from build123d import *

# Parameters (mm, degrees)
BOSS_EXTRUDE1_DEPTH      = 96
SKETCH3_W                = 68
SKETCH3_H                = 10
CUT_EXTRUDE1_DEPTH       = 96
SKETCH6_W                = 5.25
SKETCH6_H                = 36
BOSS_EXTRUDE3_DEPTH      = 7
BOSS_EXTRUDE3_DEPTH_BACK = 103
SKETCH8_W                = 5.25
SKETCH8_H                = 7
BOSS_EXTRUDE4_DEPTH      = 4
SKETCH10_W               = 5.25
SKETCH10_H               = 7
BOSS_EXTRUDE5_DEPTH      = 4
SKETCH11_W               = 96
SKETCH11_H               = 36
CUT_EXTRUDE2_DEPTH       = 101
SKETCH12_R               = 1.85
CUT_EXTRUDE3_DEPTH       = 111
SKETCH13_W               = 96
SKETCH13_H               = 3.5
CUT_EXTRUDE4_DEPTH       = 10
SKETCH14_W               = 1
SKETCH14_H               = 13.753189639
CUT_EXTRUDE5_DEPTH       = 10
SKETCH15_W               = 25
SKETCH15_H               = 24
BOSS_EXTRUDE6_DEPTH      = 5
SKETCH16_W               = 22
SKETCH16_H               = 24
CUT_EXTRUDE6_DEPTH       = 3


with BuildPart() as part:
    # Sketch1 → Boss-Extrude1 (new body)
    with BuildSketch(Plane.XY):
        Polygon((2.5, 3), (5, 3), (5, -3), (-5, -3), (-5, 3), (-2.5, 3), (-2.5, 7), (-33, 7), (-33, 15.720359308), (-29, 15.720359308), (-29, 11), (29, 11), (29, 17.148290328), (33, 17.148290328), (33, 7), (2.5, 7), align=None)
    extrude(amount=-BOSS_EXTRUDE1_DEPTH)

    # Sketch3 → Cut-Extrude1 (cut)
    with BuildSketch(Plane.ZY.offset(5)):
        with Locations((-48, 2)):
            Rectangle(SKETCH3_W, SKETCH3_H)
    extrude(amount=-CUT_EXTRUDE1_DEPTH, mode=Mode.SUBTRACT)

    # Sketch6 → Boss-Extrude3 (add, two sides)
    with BuildSketch(Plane.XY) as boss_extrude3_sk:
        with Locations((14.625, -11)):
            Rectangle(SKETCH6_W, SKETCH6_H)
    extrude(amount=BOSS_EXTRUDE3_DEPTH)
    extrude(boss_extrude3_sk.sketch, amount=-BOSS_EXTRUDE3_DEPTH_BACK)

    # Sketch8 → Boss-Extrude4 (add)
    with BuildSketch(Plane(origin=(0, 7, 0), x_dir=(1, 0, 0), z_dir=(0, 1, 0))):
        with Locations((14.625, 99.5)):
            Rectangle(SKETCH8_W, SKETCH8_H)
    extrude(amount=BOSS_EXTRUDE4_DEPTH)

    # Sketch10 → Boss-Extrude5 (add)
    with BuildSketch(Plane(origin=(0, 7, 0), x_dir=(1, 0, 0), z_dir=(0, 1, 0))):
        with Locations((14.625, -3.5)):
            Rectangle(SKETCH10_W, SKETCH10_H)
    extrude(amount=BOSS_EXTRUDE5_DEPTH)

    # Sketch11 → Cut-Extrude2 (cut)
    with BuildSketch(Plane.ZY.offset(-12)):
        with Locations((-48, -11)):
            Rectangle(SKETCH11_W, SKETCH11_H)
    extrude(amount=-CUT_EXTRUDE2_DEPTH, mode=Mode.SUBTRACT)

    # Sketch12 → Cut-Extrude3 (cut, through all)
    with BuildSketch(Plane.XY.offset(7)):
        with Locations((14.5, -25.3)):
            Circle(SKETCH12_R)
        with Locations((14.5, -9.6)):
            Circle(SKETCH12_R)
    extrude(amount=-CUT_EXTRUDE3_DEPTH, mode=Mode.SUBTRACT)

    # Sketch13 → Cut-Extrude4 (cut)
    with BuildSketch(Plane.ZY.offset(33)):
        with Locations((-48, 13.970359308)):
            Rectangle(SKETCH13_W, SKETCH13_H)
    extrude(amount=-CUT_EXTRUDE4_DEPTH, mode=Mode.SUBTRACT)

    # Sketch14 → Cut-Extrude5 (cut)
    with BuildSketch(Plane.ZY.offset(-12)):
        with Locations((0.5, 0.12340518)):
            Rectangle(SKETCH14_W, SKETCH14_H)
        with Locations((-96.5, 0.12340518)):
            Rectangle(SKETCH14_W, SKETCH14_H)
    extrude(amount=-CUT_EXTRUDE5_DEPTH, mode=Mode.SUBTRACT)

    # Sketch15 → Boss-Extrude6 (add)
    with BuildSketch(Plane.ZY.offset(33)):
        with Locations((-48, 9.610179654)):
            Rectangle(SKETCH15_W, SKETCH15_H)
    extrude(amount=BOSS_EXTRUDE6_DEPTH)

    # Sketch16 → Cut-Extrude6 (cut)
    with BuildSketch(Plane.ZY.offset(38)):
        with Locations((-48, 9.610179654)):
            Rectangle(SKETCH16_W, SKETCH16_H)
    extrude(amount=-CUT_EXTRUDE6_DEPTH, mode=Mode.SUBTRACT)


solid = part.part
Here's how the part is built. I have some questions about the finished solid (model axes, mm). A direction names the side the tool comes from. Round coordinates to 2 decimals unless told otherwise and drop trailing zeros. Loops run counter-clockwise (first coordinate to the right, second up) from the corner with the lowest first, then second, coordinate; pieces in that order, holes last.
1. If we section it at D-D on x = 23: Write out the boundary of the cut face in (y, z).
Answer list:
outline: (7, -96) - (11, -96) - (11, 0) - (7, 0) - close
2. For P1, Ø5, axis at x = 15, z = -47, coming from the -Y side; P2, Ø3, axis at y = 1, z = -6, coming from the +X side; P3, Ø11, axis at x = 0, z = -6, coming from the -Y side; P4, Ø3.5, axis at x = 14.5, y = -25.3, coming from the -Z side, each with a flat end and sliding along its axis, tell me the tip position at first contact or that it passes through.
Answer list:
P1: stops at y = 7
P2: stops at x = 5
P3: stops at y = -3
P4: passes through
3. If we section it at C-C on z = -62: Write out the boundary of the cut face in (x, y), plus the area to 3 significant figures.
Answer list:
outline: (-33, 7) - (33, 7) - (33, 17.15) - (29, 17.15) - (29, 11) - (-29, 11) - (-29, 12.22) - (-33, 12.22) - close
area: 293 mm2
4. If we section it at B-B on x = 14.5: Write out the boundary of the cut face in (y, z), plus the area to 3 significant figures.
Answer list:
outline: (-29, -103) - (-27.15, -103) - (-27.15, -96) - (-29, -96) - close; (-29, 0) - (-27.15, 0) - (-27.15, 7) - (-29, 7) - close; (-23.45, -103) - (-11.45, -103) - (-11.45, -96) - (-23.45, -96) - close; (-23.45, 0) - (-11.45, 0) - (-11.45, 7) - (-23.45, 7) - close; (-7.75, -103) - (11, -103) - (11, 7) - (-7.75, 7) - (-7.75, 0) - (-6.75, 0) - (-6.75, 1) - (7, 1) - (7, -97) - (-6.75, -97) - (-6.75, -96) - (-7.75, -96) - close
area: 813 mm2
5. If we section it at A-A on y = -9.6: Write out the boundary of the cut face in (x, z).
Answer list:
outline: (12, -103) - (12.65, -103) - (12.65, -96) - (12, -96) - close; (12, 0) - (12.65, 0) - (12.65, 7) - (12, 7) - close; (16.35, -103) - (17.25, -103) - (17.25, -96) - (16.35, -96) - close; (16.35, 0) - (17.25, 0) - (17.25, 7) - (16.35, 7) - close
6. Which directions (+Z, -Z, +X, -X, +Y, -Y) give clear straight access to the entire face, cutting with the end or side of a thin tool? Please do faces 5 (the face through (-7, 9, 0)), 6 (the face through (0, 11, -49)), 7 (the face through (-5, 0, -7)), 8 (the face through (2.5, 5, -89)), 9 (the face through (5, 0, -7)).
Answer list:
face 5: +Z, -X, +Y, -Y
face 6: +Z, -Z, +Y
face 7: +Z, -Z, -X, -Y
face 8: +Z, -Z, +X
face 9: +Z, -Z, +X, -Y
7. We'd pull the mould along X, two halves only. Please class faces 1 (the face through (15, -18, -96)), 2 (the face through (12, -9, -99)), 3 (the face through (15.354, -26.941, -99.451)), 4 (the face through (-31, 12.22, -49)): +X half, -X half, draft (parallel to the pull), parting line (faces both ways), or undercut.
Answer list:
face 1: draft
face 2: -X half
face 3: undercut
face 4: undercut
8. If I drill on line 1 along Y through (x, z) = (14.5, 5.25); line 2 along X through (y, z) = (-25, 3); line 3 along Z through (x, y) = (-12.5, 9), over which ranges is the centre line in solid material (lowest first)?
Answer list:
line 1: y = -29 to -27.15, -23.45 to -11.45, -7.75 to 11
line 2: x = 12 to 12.67, 16.33 to 17.25
line 3: z = -96 to 0
